Work out the finished part from the listing and answer in its coordinate system (mm). Coordinates: 2 decimals unless noted, no trailing zeros. Order: outer loops, then holes, each group sorted by start corner. A loop starts at its lowest first (then second) coordinate and runs counter-clockwise, first axis right, second up.
1. The part is cut by section A-A, the plane x = 109.5. Give the vertices of the cut face in (y, z) (3 decimals).
2. Find the intervals of material crossed by probe 1 along Z at (x, y) = (77.5, 2.45); probe 2 along X at (y, z) = (0.95, -84); probe 3 along Z at (x, y) = (72.5, 1.5), in increasing order.
3. A flat-ended cylindrical pin translates along its axis: pin 1 Ø20 at (x, z) = (77.01, -148.6) entering from -Y. Find the tip coordinate at first contact, or state that the pin passes through.
4. The part is cut by section D-D, the plane y = 2.4. Count the separate pieces of the cut face and the enclosed holes in it, then the cut area to 3 significant figures.
5. The part is cut by section C-C, the plane x = 72. Give the vertices of the cut face in (y, z) (3 decimals), then the cut area to 3 significant figures.
6. The part is cut by section B-B, the plane z = -62. Give the vertices of the cut face in (x, y) (3 decimals), then the cut area to 3 significant figures.
7. Determine the mould class of faces 1 (the cylindrical face through (1.91, 1.57, -71.66)), 2 (the flat face through (128, 2, -126)), 3 (the cylindrical face through (35.94, 1.57, -34.26)) for opening direction X: +X half, -X half, draft (parallel to the pull), parting line (faces both ways), or undercut.
Autodesk Inventor part; units mm, degrees
ref_plane "YZ Plane" through (0, 0, 0) normal (1, 0, 0) x (0, 1, 0)
ref_plane "XZ Plane" through (0, 0, 0) normal (0, 1, 0) x (-1, 0, 0)
ref_plane "XY Plane" through (0, 0, 0) normal (0, 0, 1) x (1, 0, 0)
sketch "Sketch1" plane through (0, 0, 0) normal (0, 1, 0) x (-1, 0, 0)
  line L0 (0, 0) -> (-165.1, 0)
  line L1 (-165.1, 0) -> (-165.1, -165.1)
  line L2 (-165.1, -165.1) -> (0, -165.1)
  line L3 (0, -165.1) -> (0, 0)
  circle A0 centre (-79.375, -79.375) radius 48.26
  line L4 (-25.4, -165.1) -> (-25.4, 0) construction
  line L5 (0, -25.4) -> (-165.1, -25.4) construction
  line L6 (0, 0) -> (-165.1, -165.1) construction
  circle A1 centre (-79.375, -79.375) radius 53.975 construction
  dimension "d0" = 96.52
  dimension "d3" = 25.4
  dimension "d4" = 25.4
  dimension "d5" = 107.95
  dimension "d24" = 165.1
extrude "Extrusion1" add sketch "Sketch1" along normal blind 3.175
sketch "Sketch2" plane through (0, 3.175, 0) normal (0, 1, 0) x (1, 0, 0)
  circle A0 centre (79.375, 79.375) radius 48.26 construction
  circle A1 centre (79.375, 79.375) radius 60.325 construction
  line L0 (0, 165.1) -> (0, 0) construction
  arc A2 (177.8, 76.2) -> (76.2, 177.8) centre (76.2, 76.2) ccw construction
  line L1 (36.7188, 36.7188) -> (122.0312, 36.7188) construction
  line L2 (122.0312, 36.7188) -> (122.0312, 122.0312) construction
  line L3 (122.0312, 122.0312) -> (36.7188, 122.0312) construction
  line L4 (36.7188, 122.0312) -> (36.7188, 36.7188) construction
  dimension "d9" = 120.65
hole "Hole1" at (36.7188, 3.175, -36.7188) at (122.0312, 3.175, -122.0312) at (122.0312, 3.175, -36.7188) at (36.7188, 3.175, -122.0312) direction (0, -1, 0) diameter 5.1594 end through all
sketch "Sketch4" plane through (0, 3.175, 0) normal (0, 1, 0) x (1, 0, 0)
  line L0 (0, 0) -> (165.1, 0)
  line L1 (0, 0) -> (25.4, 0)
  line L2 (25.4, 0) -> (25.4, 69.85)
  line L3 (25.4, 69.85) -> (0, 69.85)
  line L4 (0, 69.85) -> (0, 0)
  line L5 (25.4, 0) -> (69.85, 0)
  line L6 (69.85, 0) -> (69.85, 25.4)
  line L7 (69.85, 25.4) -> (25.4, 25.4)
  line L8 (25.4, 25.4) -> (25.4, 0)
  dimension "d26" = 25.4
  dimension "d27" = 69.85
  dimension "d28" = 44.45
  dimension "d29" = 25.4
extrude "Extrusion3" cut sketch "Sketch4" against normal through all
chamfer "Chamfer1" distance 76.2 angle 45 1 edges at (165.1, 1.5875, -165.1)
fillet "Fillet4" radius 6.35 7 edges at (165.1, 1.5875, 0) (165.1, 1.5875, -88.9) (88.9, 1.5875, -165.1) (0, 1.5875, -165.1) (0, 1.5875, -69.85) (25.4, 1.5875, -25.4) (69.85, 1.5875, 0)
sketch "Sketch5" plane through (0, 3.175, 0) normal (0, 1, 0) x (1, 0, 0)
  circle A0 centre (148.6003, 77.0066) radius 11.1125
  circle A1 centre (79.375, 79.375) radius 48.26 construction
  circle A2 centre (79.375, 79.375) radius 69.2658 construction
  circle A3 centre (136.0149, 57.9229) radius 25.4 construction
  circle A4 centre (122.0312, 36.7188) radius 2.5797 construction
  circle A5 centre (136.0149, 57.9229) radius 22.86 construction
  line L0 (122.0312, 36.7188) -> (148.6003, 77.0066) construction
  circle A6 centre (36.7188, 36.7188) radius 2.5797 construction
  circle A7 centre (122.0312, 122.0312) radius 2.5797 construction
  line L1 (36.7188, 36.7188) -> (122.0312, 122.0312) construction
  circle A8 centre (77.0066, 148.6003) radius 11.1125
  point P0 (0, 0)
  dimension "d38" = 138.5316
  dimension "d39" = 50.8
  dimension "d40" = 45.72
  dimension "d37" = 22.225
extrude "Extrusion4" cut sketch "Sketch5" against normal through all
properties part number "BottomPlate" material "Aluminum 6061"
Geometry says:
1. outline: (0, -144.5) - (3.175, -144.5) - (3.175, -117.078) - (0, -117.078) - close; (0, -41.672) - (3.175, -41.672) - (3.175, 0) - (0, 0) - close
2. probe 1: z = -165.1 to -159.7, -137.5 to -127.6, -31.15 to 0
2. probe 2: x = 0 to 31.34, 127.41 to 139.96, 157.24 to 165.1
2. probe 3: z = -165.1 to -158.76, -138.44 to -127.14, -31.61 to -1.19
3. pin 1: passes through
4. separate pieces: 1
4. enclosed holes: 7
4. area: 13,200 mm2
5. outline: (0, -165.1) - (3.175, -165.1) - (3.175, -158.521) - (0, -158.521) - close; (0, -138.68) - (3.175, -138.68) - (3.175, -127.068) - (0, -127.068) - close; (0, -31.682) - (3.175, -31.682) - (3.175, -1.587) - (0, -1.587) - close
5. area: 153 mm2
6. outline: (25.4, 0) - (34.351, 0) - (34.351, 3.175) - (25.4, 3.175) - close; (124.399, 0) - (165.1, 0) - (165.1, 3.175) - (124.399, 3.175) - close
6. area: 158 mm2
7. face 1: -X half
7. face 2: +X half
7. face 3: undercut
